from build123d import *

# Parameters (mm, degrees)
SKETCH1_W           = 99.8
SKETCH1_H           = 34
BOSS_EXTRUDE1_DEPTH = 5
SKETCH2_R           = 2.15
CUT_EXTRUDE1_DEPTH  = 5
FILLET1_R           = 2


with BuildPart() as part:
    # Sketch1 → Boss-Extrude1 (new body)
    with BuildSketch(Plane(origin=(0, 0, 0), x_dir=(1, 0, 0), z_dir=(0, 1, 0))):
        Rectangle(SKETCH1_W, SKETCH1_H)
    extrude(amount=BOSS_EXTRUDE1_DEPTH)

    # Sketch2 → Cut-Extrude1 (cut)
    with BuildSketch(Plane(origin=(0, 5, 0), x_dir=(1, 0, 0), z_dir=(0, 1, 0))):
        with Locations(Location((-43.9, 12, 0), (0, 0, 270))):
            Circle(SKETCH2_R)
        with Locations(Location((-25.9, 12, 0), (0, 0, 270))):
            Circle(SKETCH2_R)
        with Locations(Location((-43.9, -12, 0), (0, 0, 270))):
            Circle(SKETCH2_R)
        with Locations(Location((-25.9, -12, 0), (0, 0, 270))):
            Circle(SKETCH2_R)
        with Locations(Location((25.9, -12, 0), (0, 0, 90))):
            Circle(SKETCH2_R)
        with Locations(Location((43.9, -12, 0), (0, 0, 90))):
            Circle(SKETCH2_R)
        with Locations(Location((25.9, 12, 0), (0, 0, 90))):
            Circle(SKETCH2_R)
        with Locations(Location((43.9, 12, 0), (0, 0, 90))):
            Circle(SKETCH2_R)
        Polygon((-13.856406461, 0), (-6.92820323, -12), (6.92820323, -12), (13.856406461, 0), (6.92820323, 12), (-6.92820323, 12), align=None)
    extrude(amount=-CUT_EXTRUDE1_DEPTH, mode=Mode.SUBTRACT)

    # Fillet1
    fillet1_edges = [part.edges().sort_by_distance(p)[0] for p in [
        (-49.9, 2.5, -17),
        (49.9, 2.5, -17),
        (49.9, 2.5, 17),
        (-49.9, 2.5, 17),
    ]]
    fillet(fillet1_edges, radius=FILLET1_R)


solid = part.part
CAD build for the part. Positions are in the model's coordinates, mm. A direction names the side the tool comes from. Round coordinates to 2 decimals unless told otherwise and drop trailing zeros. Write each loop counter-clockwise with the first axis right and the second up, starting at its lowest first coordinate (ties: lowest second). Pieces come first, ordered by that corner, then holes.
(1) Probe line 1 along Z through (x, y) = (26, 3.3); line 2 along Z through (x, y) = (-2, 3.4); line 3 along X through (y, z) = (3.7, -10.5). List the from-to ranges inside material, lowest first.
(2) Slice it at C-C, the plane z = 8.5. Write the cut outline in (x, y), and give its area (3 significant figures).
(3) Mould opens along Z. For faces 3 (the face through (0, 3, 12)), 4 (the face through (-23.77, 2.54, 11.72)), 5 (the face through (49.3, 2.54, 16.43)), 6 (the face through (-49.33, 2.54, -16.4)) say: pulls with the +Z half, pulls with the -Z half, needs draft (parallel to the pull), parting line crosses it, or undercut.
(4) Slice it at A-A, the plane x = -25.9. Write the cut outline in (y, z).
(5) 3-axis set-ups, long thin cutter, end or side, ignore diameter. For faces 1 (the face through (10.344, 2.535, 6.084)), 2 (the face through (-1, 2, -17)): which of +Z, -Z, +X, -X, +Y, -Y reach the whole face in a straight line?
(6) Slice it at B-B, the plane y = 1.8. Count the separate pieces of the cut face and the enclosed holes in it, and give its area (3 significant figures).
From the geometry:
1. line 1: z = -17 to -14.15, -9.85 to 9.85, 14.15 to 17
1. line 2: z = -17 to -12, 12 to 17
1. line 3: x = -49.9 to -45.44, -42.36 to -27.44, -24.36 to -7.79, 7.79 to 24.36, 27.44 to 42.36, 45.44 to 49.9
2. outline: (-49.9, 0) - (-8.95, 0) - (-8.95, 5) - (-49.9, 5) - close; (8.95, 0) - (49.9, 0) - (49.9, 5) - (8.95, 5) - close
2. area: 410 mm2
3. face 3: undercut
3. face 4: undercut
3. face 5: pulls with the +Z half
3. face 6: pulls with the -Z half
4. outline: (0, -17) - (5, -17) - (5, -14.15) - (0, -14.15) - close; (0, -9.85) - (5, -9.85) - (5, 9.85) - (0, 9.85) - close; (0, 14.15) - (5, 14.15) - (5, 17) - (0, 17) - close
5. face 1: +Y, -Y
5. face 2: -Z, +X, -X, +Y, -Y
6. separate pieces: 1
6. enclosed holes: 9
6. area: 2,770 mm2
